from build123d import *

# Parameters (mm, degrees)
SKETCH_1_W          = 34.5
SKETCH_1_H          = 25.5
EXTRUDE_1_DEPTH     = 5
SKETCH_5_W          = 32.5
SKETCH_5_H          = 3.3
CUT_EXTRUDE_1_DEPTH = 23.025553342
SKETCH_7_R          = 1.25
CUT_EXTRUDE_2_DEPTH = 38.118896805


with BuildPart() as part:
    # 草图1 → 凸台-拉伸1 (new body)
    with BuildSketch(Plane(origin=(0, 0, 0), x_dir=(1, 0, 0), z_dir=(0, 1, 0))):
        Rectangle(SKETCH_1_W, SKETCH_1_H)
    extrude(amount=EXTRUDE_1_DEPTH)

    # 草图5 → 切除-拉伸1 (cut, through all)
    with BuildSketch(Plane.XZ):
        with Locations((0, 8)):
            Rectangle(SKETCH_5_W, SKETCH_5_H)
    extrude(amount=-CUT_EXTRUDE_1_DEPTH, mode=Mode.SUBTRACT)

    # 草图7 → 切除-拉伸2 (cut, through all)
    with BuildSketch(Plane(origin=(17.25, 0, 0), x_dir=(0, 0, -1), z_dir=(1, 0, 0))):
        with Locations((-8, 2.5)):
            Circle(SKETCH_7_R)
    extrude(amount=-CUT_EXTRUDE_2_DEPTH, mode=Mode.SUBTRACT)

    # 草图8 → M2x0.4 螺纹孔1 (revolve, cut)
    with BuildSketch(Plane(origin=(0, 2.5, -12.75), x_dir=(0, 1, 0), z_dir=(1, 0, 0))):
        Polygon((0, 0), (0, 5.680688495), (0.8, 5.2), (0.8, 0), align=None)
    m2x0_4_1 = revolve(axis=Axis((0, 2.5, -19.1), (0, 0, 1)), mode=Mode.SUBTRACT)

    # 镜向1: M2x0.4 螺纹孔1 across plane
    add(m2x0_4_1.mirror(Plane.XY), mode=Mode.SUBTRACT)


solid = part.part
CAD build for the part. Positions are in the model's coordinates, mm. A direction names the side the tool comes from. Coordinates: 2 decimals unless noted, no trailing zeros. Loops run counter-clockwise (first coordinate to the right, second up) from the corner with the lowest first, then second, coordinate; pieces in that order, holes last. Notation, with made-up numbers: (74, 9.25) -> (103, 9.25) arc R22 ccw to (103, 27.25) -> close; hole circle Ø9 at (-30, 49.5). An arc over 180 degrees is marked (long way). One line per item, written item: value.
1. Pull direction Y, two halves, no side cores. Call faces 1 (the face through (0, 0, 0)), 2 (the face through (17.25, 2, 0)), 3 (the face through (0.78, 2.33, 11.22)): pulls with the +Y half, pulls with the -Y half, needs draft (parallel to the pull), parting line crosses it, or undercut.
Answers:
face 1: pulls with the -Y half
face 2: needs draft
face 3: undercut
2. Which spindle directions (+Z, -Z, +X, -X, +Y, -Y) get a long thin tool onto all of the face, cutting with end or side? Do faces 4 (the face through (16.76, 2.55, 9.25)), 5 (the face through (16.25, 1, 7)), 6 (the face through (0.78, 2.33, -10.19)). Say none if no direction does.
Answers:
face 4: +X, -X
face 5: +Y, -Y
face 6: -Z
3. Slice it at B-B on x = -9. Write the cut outline in (y, z), and give its area (3 significant figures).
Answers:
outline: (0, -12.75) -> (5, -12.75) -> (5, 6.35) -> (0, 6.35) -> close; (0, 9.65) -> (5, 9.65) -> (5, 12.75) -> (0, 12.75) -> close
area: 111 mm^2
4. Drill centre lines: line 1 (X direction, y = 2.35, z = 6.5); line 2 (Y direction, x = 0, z = -8.8); line 3 (Y direction, x = 16.95, z = 8). Where is each one in solid material? Low to high. Write a range as [from, to].
Answers:
line 1: x = [-17.25, -16.25], [16.25, 17.25]
line 2: y = [0, 1.7], [3.3, 5]
line 3: y = [0, 1.25], [3.75, 5]
5. Flat gauge pins, fed straight in: P1, Ø1.3, axis at x = 0, y = 2.5, coming from the +Z side; P2, Ø3, axis at x = 4, z = -6.5, coming from the -Y side; P3, Ø1.7, axis at y = 2.5, z = 8, coming from the -X side (1 decimal). Where does each tip first touch, or does it go through?
Answers:
P1: stops at z = 6.35
P2: stops at y = 0
P3: passes through
6. Slice it at A-A on z = 8. Write the cut outline in (x, y), and give its area (3 significant figures).
Answers:
outline: (-17.25, 0) -> (-16.25, 0) -> (-16.25, 1.25) -> (-17.25, 1.25) -> close; (-17.25, 3.75) -> (-16.25, 3.75) -> (-16.25, 5) -> (-17.25, 5) -> close; (16.25, 0) -> (17.25, 0) -> (17.25, 1.25) -> (16.25, 1.25) -> close; (16.25, 3.75) -> (17.25, 3.75) -> (17.25, 5) -> (16.25, 5) -> close
area: 5.00 mm^2
7. Slice it at C-C on y = 0.6. Write the cut outline in (x, z), and give its area (4 significant figures).
Answers:
outline: (-17.25, -12.75) -> (17.25, -12.75) -> (17.25, 12.75) -> (-17.25, 12.75) -> close; hole (-16.25, 6.35) -> (16.25, 6.35) -> (16.25, 9.65) -> (-16.25, 9.65) -> close
area: 772.5 mm^2
